```python
from build123d import *

# Parameters (mm, degrees)
SKETCH1_W           = 25.4
SKETCH1_H           = 1.5875
BOSS_EXTRUDE1_DEPTH = 0.79375
BOSS_EXTRUDE2_DEPTH = 482.6


with BuildPart() as part:
    # Sketch1 → Boss-Extrude1 (new body)
    # profile 1 of 2: a face of its own
    with BuildSketch(Plane(origin=(-94.488, 0, 0), x_dir=(0, -1, 0), z_dir=(-1, 0, 0))):
        Polygon((136.525, -196.85), (111.125, -196.85), (111.125, -203.2), (85.725, -203.2), (85.725, -196.85), (60.325, -196.85), (60.325, -682.625), (85.725, -682.625), (85.725, -679.45), (111.125, -679.45), (111.125, -682.625), (136.525, -682.625), align=None)
        with Locations((98.425, -456.40625)):
            Rectangle(SKETCH1_W, SKETCH1_H, mode=Mode.SUBTRACT)
    # profile 2 of 2: a face of its own
    with BuildSketch(Plane(origin=(-94.488, 0, 0), x_dir=(0, -1, 0), z_dir=(-1, 0, 0))):
        with BuildLine():
            Line((149.225, -203.2), (136.525, -203.2))
            Line((136.525, -203.2), (136.525, -290.406498707))
            ThreePointArc((136.525, -290.406498707), (137.30121982, -286.034603668), (139.534994681, -282.197126202))
            Line((139.534994681, -282.197126202), (184.118202659, -229.57294303))
            ThreePointArc((184.118202659, -229.57294303), (185.23509009, -227.654204297), (185.6232, -225.468256778))
            Line((185.6232, -225.468256778), (185.6232, -203.2))
            Line((185.6232, -203.2), (168.275, -203.2))
            Line((168.275, -203.2), (168.275, -196.85))
            Line((168.275, -196.85), (149.225, -196.85))
            Line((149.225, -196.85), (149.225, -203.2))
        make_face()
    extrude(amount=-BOSS_EXTRUDE1_DEPTH)

    # Sketch4 → Boss-Extrude2 (add)
    with BuildSketch(Plane(origin=(0, 0, -679.45), x_dir=(-1, 0, 0), z_dir=(0, 0, -1))):
        with BuildLine():
            Line((97.166105032, -116.822884411), (94.488, -136.525))
            Line((94.488, -136.525), (94.488, -114.25313135))
            Line((94.488, -114.25313135), (94.488, -111.125))
            Line((94.488, -111.125), (94.488, -108.585))
            ThreePointArc((94.488, -108.585), (95.231948776, -110.381051224), (97.028, -111.125))
            Line((97.028, -111.125), (113.793536469, -111.125))
            ThreePointArc((113.793536469, -111.125), (114.50064325, -111.417893219), (114.793536469, -112.125))
            Line((114.793536469, -112.125), (114.793536469, -113.625))
            ThreePointArc((114.793536469, -113.625), (114.50064325, -114.332106781), (113.793536469, -114.625))
            Line((113.793536469, -114.625), (99.682959601, -114.625))
            ThreePointArc((99.682959601, -114.625), (98.012237242, -115.251812399), (97.166105032, -116.822884411))
        make_face()
    extrude(amount=-BOSS_EXTRUDE2_DEPTH)


solid = part.part
```
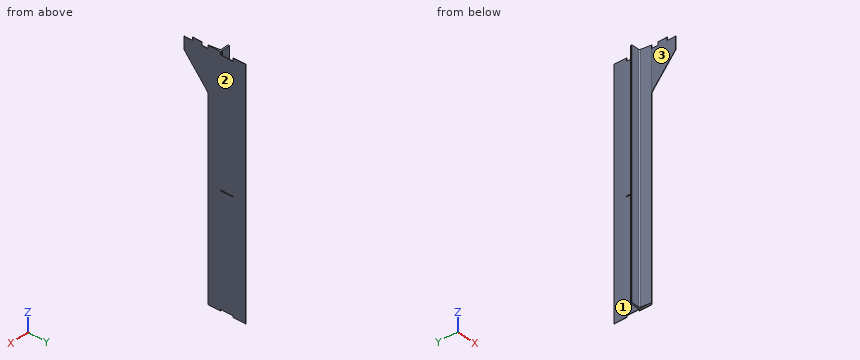
Input: part model. Units: mm. Frame: model coordinates. Face numbers are marked on the shaded views. A direction names the side the tool comes from. Give positions to 0.01 mm unless a question says otherwise; leave off trailing zeros. Order: outer loops, then holes, each group sorted by start corner. A loop starts at its lowest first (then second) coordinate and runs counter-clockwise, first axis right, second up.
1. Pin query (flat end, axial travel): pin 1 (0.9 mm diameter, centred on x = -94, z = -199, fed in from -Y) (3 decimals); pin 2 (10.5 mm diameter, centred on x = -104, y = -118.5, fed in from -Z); pin 3 (2 mm diameter, centred on y = -76, z = -393, fed in from -X). Return the tip coordinate at first contact, or that it passes through.
Derived:
pin 1: stops at y = -168.275
pin 2: stops at z = -679.45
pin 3: stops at x = -94.49
2. Section C-C on y = -129. Return the cut outline in (x, z) (3 decimals).
Derived:
outline: (-95.511, -679.45) - (-94.488, -679.45) - (-94.488, -682.625) - (-93.694, -682.625) - (-93.694, -196.85) - (-95.511, -196.85) - close
3. Section D-D on x = -107.25. Return the cut outline in (y, z) (3 decimals).
Derived:
outline: (-114.625, -679.45) - (-111.125, -679.45) - (-111.125, -196.85) - (-114.625, -196.85) - close
4. Material intervals for L1, parallel to X at y = -97, z = -619; L2, parallel to Y at x = -100, z = -370 (3 decimals); L3, parallel to X at y = -117, z = -548.5, sorted ascending.
Derived:
L1: x = -94.49 to -93.69
L2: y = -114.625 to -111.125
L3: x = -97.14 to -93.69
5. Section A-A on y = -103. Return the cut outline in (x, z), and give its area (3 significant figures).
Derived:
outline: (-94.49, -679.45) - (-93.69, -679.45) - (-93.69, -457.2) - (-94.49, -457.2) - close; (-94.49, -455.61) - (-93.69, -455.61) - (-93.69, -203.2) - (-94.49, -203.2) - close
area: 377 mm2
6. Reachability of the marked faces 1, 2 and 3 from +Z, -Z, +X, -X, +Y, -Y: full face, straight path, thin tool, end or side. Return the list, or none.
Derived:
face 1: +Z, -Z, -X, +Y
face 2: +Z, -Z, +X, +Y, -Y
face 3: +Z, -Z, -X, -Y
7. Section B-B on z = -589. Return the cut outline in (x, y) (3 decimals), and give its area (3 significant figures).
Derived:
outline: (-114.794, -113.625) arc R1 ccw to (-113.794, -114.625) - (-99.683, -114.625) arc R2.54 cw to (-97.166, -116.823) - (-94.488, -136.525) - (-93.694, -136.525) - (-93.694, -60.325) - (-94.488, -60.325) - (-94.488, -108.585) arc R2.54 cw to (-97.028, -111.125) - (-113.794, -111.125) arc R1 ccw to (-114.794, -112.125) - close
area: 166 mm2
